Can you work these out from the model? Positions are in its coordinate system, mm. Give positions to 0.01 mm unless a question says otherwise; leave off trailing zeros. Order: outer loops, then holes, each group sorted by start corner. A loop starts at its lowest first (then second) coordinate and runs counter-clockwise, first axis right, second up. Notation, with made-up numbers: (76.25, 28.25) - (129.25, 28.25) arc R21 ccw to (129.25, 54.25) - close; hole circle Ø8 at (-23, -16.75). An arc over 180 degrees is marked (long way). Answer as CSV lines item,"result".
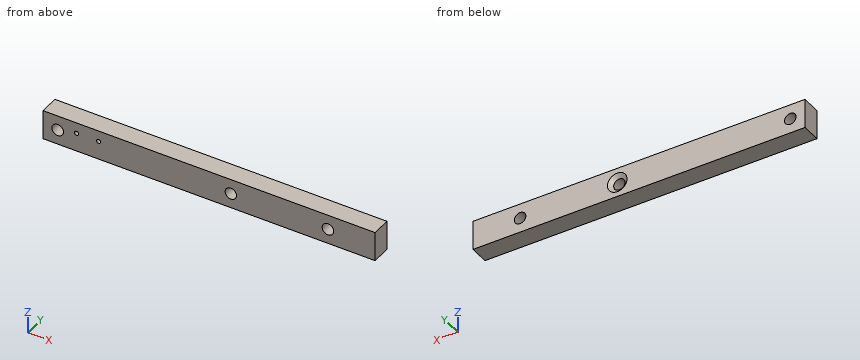
```python
from build123d import *

# Parameters (mm, degrees)
SKETCH1_W                                         = 143.256
SKETCH1_H                                         = 12.7
BOSS_EXTRUDE1_DEPTH                               = 8.255
CSK_FOR_8_FLAT_HEAD_MACHINE_SCREW_100_D           = 4.9149
CSK_FOR_8_FLAT_HEAD_MACHINE_SCREW_100_CSINK_D     = 8.4328
CSK_FOR_8_FLAT_HEAD_MACHINE_SCREW_100_CSINK_ANGLE = 100
TAP_DRILL_FOR_2_56_TAP2_D                         = 1.778
TAP_DRILL_FOR_2_56_TAP2_DEPTH                     = 6.35
TAP_DRILL_FOR_2_56_TAP2_TIP                       = 0.53416509
TAP_DRILL_FOR_M6X1_0_TAP1_D                       = 5


with BuildPart() as part:
    # Sketch1 → Boss-Extrude1 (new body)
    with BuildSketch(Plane(origin=(0, 0, 0), x_dir=(1, 0, 0), z_dir=(0, 1, 0))):
        with Locations((7.131792208, 4.399367965)):
            Rectangle(SKETCH1_W, SKETCH1_H)
    extrude(amount=BOSS_EXTRUDE1_DEPTH)

    # CSK for #8 Flat Head Machine Screw (100)1 (through all)
    with Locations(Plane(origin=(0, 8.255, 0), x_dir=(1, 0, 0), z_dir=(0, 1, 0))):
        with Locations((16.529792208, 4.399367965)):
            CounterSinkHole(CSK_FOR_8_FLAT_HEAD_MACHINE_SCREW_100_D / 2, CSK_FOR_8_FLAT_HEAD_MACHINE_SCREW_100_CSINK_D / 2, counter_sink_angle=CSK_FOR_8_FLAT_HEAD_MACHINE_SCREW_100_CSINK_ANGLE)

    # Tap Drill for #2-56 Tap2
    with Locations(Plane(origin=(0, 0, 0), x_dir=(-1, 0, 0), z_dir=(0, -1, 0))):
        with Locations((50.027522326, 2.748367965), (40.502522326, 2.748367965)):
            Hole(TAP_DRILL_FOR_2_56_TAP2_D / 2, depth=TAP_DRILL_FOR_2_56_TAP2_DEPTH)
            with Locations((0, 0, -(TAP_DRILL_FOR_2_56_TAP2_DEPTH + TAP_DRILL_FOR_2_56_TAP2_TIP / 2))):  # 118° drill point
                Cone(0, TAP_DRILL_FOR_2_56_TAP2_D / 2, TAP_DRILL_FOR_2_56_TAP2_TIP, mode=Mode.SUBTRACT)

    # Tap Drill for M6x1.0 Tap1 (through all)
    with Locations(Plane(origin=(0, 8.255, 0), x_dir=(1, 0, 0), z_dir=(0, 1, 0))):
        with Locations((58.439792208, 4.399367965), (-58.146207792, 4.399367965)):
            Hole(TAP_DRILL_FOR_M6X1_0_TAP1_D / 2)


solid = part.part
```
1) I'm going to push flat-ended pins straight in: P1, Ø4, axis at x = -58.15, z = -4.4, coming from the -Y side; P2, Ø3, axis at x = 35.5, z = -1.5, coming from the -Y side. Where does each tip first touch, or does it pass through?
Answer block:
P1,"through"
P2,"y = 0"
2) I want a section at A-A on y = 3. Write out the boundary of the cut face in (x, z).
Answer block:
outline,"(-64.5, -10.75) - (78.76, -10.75) - (78.76, 1.95) - (-64.5, 1.95) - close; hole circle Ø5 at (-58.15, -4.4); hole circle Ø1.78 at (-50.03, -2.75); hole circle Ø1.78 at (-40.5, -2.75); hole circle Ø4.91 at (16.53, -4.4); hole circle Ø5 at (58.44, -4.4)"
3) I need wall thicknesses on line 1 along X through (y, z) = (3.5, -4.75); line 2 along X through (y, z) = (7, -2.75); line 3 along X through (y, z) = (0.75, -2.75). Which ranges of each line are inside material? Lowest first, please. Write a range as [from, to].
Answer block:
line 1,"[-64.5, -60.62], [-55.67, 14.1], [18.96, 55.96], [60.92, 78.76]"
line 2,"[-64.5, -60.02], [-56.27, 14.37], [18.69, 56.56], [60.32, 78.76]"
line 3,"[-64.5, -60.02], [-56.27, -50.92], [-49.14, -41.39], [-39.61, 14.71], [18.35, 56.56], [60.32, 78.76]"
